Here's how the part is built. I have some questions about the finished solid (model axes, mm). Face numbers are marked on the shaded views. Give positions to 0.01 mm unless a question says otherwise; leave off trailing zeros. Write each loop counter-clockwise with the first axis right and the second up, starting at its lowest first coordinate (ties: lowest second). Pieces come first, ordered by that corner, then holes. Notation, with made-up numbers: (72, 21.25) - (88, 21.25) arc R23 ccw to (88, 58.25) - close; hole circle Ø9 at (2, -30.75). An arc over 180 degrees is marked (long way). One line per item, written item: value. Start each with the question number.
1) Imagine slicing it at D-D on y = 9.75. Write out the boundary of the cut face in (x, z).
2) Imagine slicing it at A-A on z = 0. Write out the boundary of the cut face in (x, y).
3) Imagine slicing it at C-C on y = 1.25. Write out the boundary of the cut face in (x, z).
4) We'd pull the mould along Z, two halves only. Please class the marked faces 1, 2 and 3: +Z half, -Z half, draft (parallel to the pull), parting line (faces both ways), or undercut.
5) Imagine slicing it at B-B on x = 30. Write out the boundary of the cut face in (y, z), plus the area to 3 significant figures.
6) I'm going to push a flat-ended pin straight in: P1, Ø17.5, axis at x = -1, z = -3, coming from the -Y side. Where does the tip first touch, or does it pass through?
7) Please list where these lines run through material, in increasing order: L1, parallel to X at y = 10.5, z = 0; L2, parallel to X at y = 4.5, z = 0; L3, parallel to Y at x = -4, z = 6.5. Write a range as [from, to].
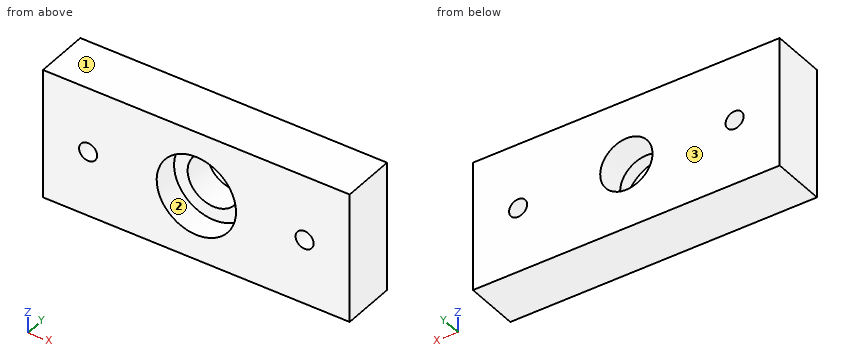
from build123d import *

# Parameters (mm, degrees)
SKETCH1_W           = 85
SKETCH1_H           = 36
SKETCH1_R           = 7.25
SKETCH1_R_2         = 2.5
BOSS_EXTRUDE1_DEPTH = 15
SKETCH2_R           = 11
CUT_EXTRUDE1_DEPTH  = 7


with BuildPart() as part:
    # Sketch1 → Boss-Extrude1 (new body)
    with BuildSketch(Plane(origin=(0, 0, 0), x_dir=(1, 0, 0), z_dir=(0, 1, 0))):
        Rectangle(SKETCH1_W, SKETCH1_H)
        with Locations(Location((0, 0, 0), (0, 0, 270))):
            Circle(SKETCH1_R, mode=Mode.SUBTRACT)
        with Locations(Location((-30, 0, 0), (0, 0, 270))):
            Circle(SKETCH1_R_2, mode=Mode.SUBTRACT)
        with Locations(Location((30, 0, 0), (0, 0, 270))):
            Circle(SKETCH1_R_2, mode=Mode.SUBTRACT)
    extrude(amount=BOSS_EXTRUDE1_DEPTH)

    # Sketch2 → Cut-Extrude1 (cut)
    with BuildSketch(Plane(origin=(0, 0, 0), x_dir=(1, 0, 0), z_dir=(0, 1, 0))):
        with Locations(Location((0, 0, 0), (0, 0, 270))):
            Circle(SKETCH2_R)
    extrude(amount=CUT_EXTRUDE1_DEPTH, mode=Mode.SUBTRACT)


solid = part.part
Numbers:
1. outline: (-42.5, -18) - (42.5, -18) - (42.5, 18) - (-42.5, 18) - close; hole circle Ø5 at (-30, 0); hole circle Ø14.5 at (0, 0); hole circle Ø5 at (30, 0)
2. outline: (-42.5, 0) - (-32.5, 0) - (-32.5, 15) - (-42.5, 15) - close; (-27.5, 0) - (-11, 0) - (-11, 7) - (-7.25, 7) - (-7.25, 15) - (-27.5, 15) - close; (7.25, 7) - (11, 7) - (11, 0) - (27.5, 0) - (27.5, 15) - (7.25, 15) - close; (32.5, 0) - (42.5, 0) - (42.5, 15) - (32.5, 15) - close
3. outline: (-42.5, -18) - (42.5, -18) - (42.5, 18) - (-42.5, 18) - close; hole circle Ø5 at (-30, 0); hole circle Ø22 at (0, 0); hole circle Ø5 at (30, 0)
4. face 1: +Z half
4. face 2: undercut
4. face 3: draft
5. outline: (0, -18) - (15, -18) - (15, -2.5) - (0, -2.5) - close; (0, 2.5) - (15, 2.5) - (15, 18) - (0, 18) - close
5. area: 465 mm^2
6. P1: y = 0
7. L1: [-42.5, -32.5], [-27.5, -7.25], [7.25, 27.5], [32.5, 42.5]
7. L2: [-42.5, -32.5], [-27.5, -11], [11, 27.5], [32.5, 42.5]
7. L3: [7, 15]
